Build history of the part. All positions in model axes, mm. A direction names the side the tool comes from. Round coordinates to 2 decimals unless told otherwise and drop trailing zeros. Write each loop counter-clockwise with the first axis right and the second up, starting at its lowest first coordinate (ties: lowest second). Pieces come first, ordered by that corner, then holes. Notation, with made-up numbers: (5, 1.25) -> (12, 1.25) arc R18 cw to (12, 6.25) -> close; hole circle Ø2 at (-12, 53). An arc over 180 degrees is marked (long way). Answer as CSV lines item,"result".
Autodesk Inventor part; units mm, degrees
ref_plane "YZ Plane" through (0, 0, 0) normal (1, 0, 0) x (0, 1, 0)
ref_plane "XZ Plane" through (0, 0, 0) normal (0, 1, 0) x (-1, 0, 0)
ref_plane "XY Plane" through (0, 0, 0) normal (0, 0, 1) x (1, 0, 0)
sketch "Sketch1" plane through (0, 0, 0) normal (0, 0, 1) x (1, 0, 0)
  line L0 (-14.3446, 13.462) -> (14.3446, 13.462)
  line L1 (14.3446, 13.462) -> (14.3446, -13.462)
  line L2 (14.3446, -13.462) -> (-14.3446, -13.462)
  line L3 (-14.3446, -13.462) -> (-14.3446, 13.462)
  line L4 (-14.3446, 13.462) -> (14.3446, -13.462) construction
  line L5 (14.3446, 13.462) -> (-14.3446, -13.462) construction
  point P0 (0, 0)
  dimension "d0" = 28.6893
  dimension "d1" = 26.924
ref_plane "Work Plane1" through (0, 0, 0) normal (0, 0, -1) x (-1, 0, 0)
sketch "Sketch2" plane through (0, 0, 0) normal (0, 0, -1) x (-1, 0, 0)
  circle A0 centre (0, 0) radius 25.4
  dimension "d4" = 50.8
extrude "Extrusion2" add sketch "Sketch2" against normal blind 6.35
extrude "Extrusion3" cut sketch "Sketch1" along normal through all
sketch "Sketch3" plane through (0, 0, 0) normal (0, 0, 1) x (1, 0, 0)
  line L0 (-14.3446, -13.462) -> (14.3446, -13.462)
  line L1 (-14.3446, 13.462) -> (-14.3446, -13.462)
  line L2 (14.3446, 13.462) -> (-14.3446, 13.462)
  line L3 (14.3446, -13.462) -> (14.3446, 13.462)
  line L4 (-14.3446, 13.462) -> (-14.3446, -13.462)
  line L5 (-14.3446, -13.462) -> (14.3446, -13.462)
  line L6 (14.3446, -13.462) -> (14.3446, 13.462)
  line L7 (14.3446, 13.462) -> (-14.3446, 13.462)
  circle A0 centre (0, 0) radius 25.4
  line L8 (-35.56, 0) -> (35.56, 0)
  line L9 (0, -35.56) -> (0, 35.56)
  line L10 (14.3446, 13.462) -> (-14.3446, 13.462)
  line L11 (-14.3446, -13.462) -> (14.3446, -13.462)
  line L12 (14.3446, -13.462) -> (14.3446, 13.462)
  line L13 (14.3446, 13.462) -> (-14.3446, 13.462)
  line L14 (-14.3446, 13.462) -> (-14.3446, -13.462)
  line L15 (-14.3446, -13.462) -> (14.3446, 13.462) construction
  line L16 (14.3446, -13.462) -> (-14.3446, 13.462) construction
  line L17 (14.3446, 13.462) -> (-14.3446, 13.462)
  line L18 (-14.3446, -13.462) -> (14.3447, -13.462)
  line L19 (14.3447, -13.462) -> (14.3446, 13.462)
  line L20 (14.3446, 13.462) -> (-14.3446, 13.462)
  line L21 (-14.3446, 13.462) -> (-14.3446, -13.462)
  line L22 (-14.3446, -13.462) -> (14.3446, 13.462) construction
  line L23 (14.3447, -13.462) -> (-14.3446, 13.462) construction
  line L24 (14.3446, -13.462) -> (14.3446, 13.462)
extrude "Extrusion4" add sketch "Sketch3" along normal blind 0.1524 contours L1 L8 L9 L0 | L9 L8 L3 L0 | L1 L2 L9 L8 | L9 L2 L3 L8
pattern_linear "Rectangular Pattern1" [suppressed]
sketch "Sketch4" plane through (0, 0, 0) normal (0, 0, 1) x (1, 0, 0)
  circle A0 centre (0, 0) radius 25.4
  line L0 (-35.56, 0) -> (35.56, 0)
  line L1 (0, -35.56) -> (0, 35.56)
  line L2 (-14.3446, -13.462) -> (14.3446, -13.462)
  line L3 (13.5954, 13.462) -> (13.5954, -13.462)
  line L4 (-12.1856, -13.462) -> (13.5954, -13.462)
  line L5 (13.5954, -13.462) -> (13.5954, -0.254)
  line L6 (13.5954, -0.254) -> (-12.1857, -0.254)
  line L7 (-12.1857, -0.254) -> (-12.1856, -13.462)
  line L8 (13.2144, 13.462) -> (13.5954, 13.462)
  line L9 (10.6744, 13.462) -> (11.0554, 13.462)
  line L10 (8.1344, 13.462) -> (8.5154, 13.462)
  line L11 (5.5944, 13.462) -> (5.9754, 13.462)
  line L12 (3.0544, 13.462) -> (3.4354, 13.462)
  line L13 (0.5144, 13.462) -> (0.8954, 13.462)
  line L14 (-2.0256, 13.462) -> (-1.6446, 13.462)
  line L15 (-4.5656, 13.462) -> (-4.1846, 13.462)
  line L16 (-7.1056, 13.462) -> (-6.7246, 13.462)
  line L17 (-9.6456, 13.462) -> (-9.2646, 13.462)
  line L18 (-12.1856, 13.462) -> (-11.8046, 13.462)
  line L19 (-12.1856, 13.462) -> (-11.8046, 13.462)
  line L20 (-12.1856, 13.462) -> (13.5954, 13.462)
  line L21 (13.5954, 13.462) -> (13.5954, 0.254)
  line L22 (13.5954, 0.254) -> (-12.1857, 0.254)
  line L23 (-12.1857, 0.254) -> (-12.1856, 13.462)
  point P0 (-11.8046, -13.462)
  dimension "d15" = 0.254
extrude "Extrusion5" [suppressed]
sketch "Sketch5" plane through (0, 0, 0) normal (0, 0, -1) x (-1, 0, 0)
  circle A0 centre (0, 0) radius 25.4
  line L0 (35.56, 0) -> (-35.56, 0)
  line L1 (0, -35.56) -> (0, 35.56)
  circle A1 centre (11.9952, -2.794) radius 0.5
  point P0 (11.9952, -0.254)
  dimension "d18" = 1
extrude "Extrusion6" cut sketch "Sketch5" against normal through all contours A1
pattern_linear "Rectangular Pattern2" count 6 spacing 5.08 along (1, 0, 0) of "Extrusion6"
mirror "Mirror1" about plane through (0, 0, 0) normal (0, 1, 0) of "Extrusion6", "Rectangular Pattern2"
sketch "Sketch6" plane through (0, 0, 0) normal (0, 0, -1) x (-1, 0, 0)
  point P0 (0, 0)
equation "\"BendRadius\" = Thickness"
equation "\"BendReliefWidth\" = Thickness"
equation "\"BendReliefDepth\" = 0.5 * Thickness"
equation "\"CornerReliefSize\" = 4 * Thickness"
equation "\"MinimumRemnant\" = 2 * Thickness"
equation "\"TransitionRadius\" = BendRadius"
equation "\"JacobiRadiusSize\" = BendRadius"
equation "\"GapSize\" = Thickness"
properties part number "_3DPrint"
1. Drop flat-ended pins along their axis: pin 1 Ø2 at (y, z) = (10, 1.5) entering from -X; pin 2 Ø1.9 at (x, z) = (-3, 4) entering from -Y; pin 3 Ø13.5 at (x, y) = (-2, -1) entering from +Z. Give the stop position or say it passes through.
Results found:
pin 1,"stops at x = -23.75"
pin 2,"stops at y = -25.32"
pin 3,"stops at z = 0.15"
2. Cut at C-C, the plane y = 0. Write the cut outline in (x, z).
Results found:
outline,"(-25.4, 0) -> (25.4, 0) -> (25.4, 6.35) -> (14.34, 6.35) -> (14.34, 0.15) -> (-14.34, 0.15) -> (-14.34, 6.35) -> (-25.4, 6.35) -> close"
3. Cut at D-D, the plane y = 19.5. Write the cut outline in (x, z), then the cut area to 3 significant figures.
Results found:
outline,"(-16.28, 0) -> (16.28, 0) -> (16.28, 6.35) -> (-16.28, 6.35) -> close"
area,"207 mm2"
4. Probe line 1 along X through (y, z) = (-0.5, 2.5); line 2 along Y through (x, z) = (4, 3.75); line 3 along Z through (x, y) = (-3.5, 6). List the from-to ranges inside material, lowest first.
Results found:
line 1,"x = -25.4 to -14.34, 14.34 to 25.4"
line 2,"y = -25.08 to -13.46, 13.46 to 25.08"
line 3,"z = 0 to 0.15"
5. Cut at B-B, the plane z = 1. Write the cut outline in (x, y).
Results found:
outline,"circle Ø50.8 at (0, 0); hole (-14.34, -13.46) -> (14.34, -13.46) -> (14.34, 13.46) -> (-14.34, 13.46) -> close"
6. Mould opens along Y. For faces 1 (the flat face through (0, -13.462, 3)), 2 (the flat face through (0, 0, 0)), 3 (the cylindrical face through (5.506, -24.796, 3.131)) say: +Y half, -Y half, draft (parallel to the pull), parting line (faces both ways), or undercut.
Results found:
face 1,"undercut"
face 2,"draft"
face 3,"parting line"
7. Which spindle directions (+Z, -Z, +X, -X, +Y, -Y) get a long thin tool onto all of the face, cutting with end or side? Do faces 4 (the flat face through (0, -17, 6.35)), 5 (the flat face through (-14.345, 0, 3)). Say none if no direction does.
Results found:
face 4,"+Z, +X, -X, +Y, -Y"
face 5,"+Z"
8. Cut at A-A, the plane x = 0. Write the cut outline in (y, z).
Results found:
outline,"(-25.4, 0) -> (25.4, 0) -> (25.4, 6.35) -> (13.46, 6.35) -> (13.46, 0.15) -> (-13.46, 0.15) -> (-13.46, 6.35) -> (-25.4, 6.35) -> close"
